Here's how the part is built. I have some questions about the finished solid (model axes, mm). A direction names the side the tool comes from. Round coordinates to 2 decimals unless told otherwise and drop trailing zeros. Order: outer loops, then holes, each group sorted by start corner. A loop starts at its lowest first (then second) coordinate and runs counter-clockwise, first axis right, second up. Notation, with made-up numbers: M 84,27 L 96,27 A22 ccw 96,38 Z; hole C 45.25,-25 d8. An arc over 180 degrees is marked long. Write each question's results on one line, items separated by ' | '. Start each with the question number.
```python
from build123d import *

# Parameters (mm, degrees)
F1_DEPTH = 12.7
F3_DEPTH = 25.4
F4_R     = 1.685949
F5_DEPTH = 25.4


with BuildPart() as f1:
    # F0 (on Front) → F1 (new body)
    with BuildSketch(Plane.XZ):
        Polygon((6.618203, -46.038546), (-16.379258, 0), (-39.209124, -45.537699), (-89.660898, -53.551219), (-53.232785, -89.361645), (-61.747152, -139.553732), (-16.671093, -115.906432), (28.655386, -139.553732), (20.14102, -89.361645), (56.902383, -53.551219), align=None)
    extrude(amount=F1_DEPTH)

    # F2 (on face) → F3 (cut)
    with BuildSketch(Plane.XZ.offset(12.7)):
        Polygon((3.150909, -52.012134), (-16.268918, -10.524325), (-34.585346, -52.012134), (-70.335478, -56.646414), (-44.074576, -82.686633), (-51.136333, -121.526286), (-16.379258, -103.871897), (18.819179, -126.60192), (10.654025, -86.879551), (38.901042, -59.073891), align=None)
    extrude(amount=-F3_DEPTH, mode=Mode.SUBTRACT)

    # F4 (on face) → F5 (cut)
    with BuildSketch(Plane.XZ.offset(12.7)):
        with Locations((-80.045395, -56.205053)):
            Circle(F4_R)
    extrude(amount=-F5_DEPTH, mode=Mode.SUBTRACT)


solid = f1.part
```
(1) I want a section at D-D on x = 42.5. Write out the boundary of the cut face in (y, z), and give its area (3 significant figures).
(2) I want a section at A-A on z = -19. Write out the boundary of the cut face in (x, y), and give its area (3 significant figures).
(3) I'm going to push flat-ended pins straight in: pin 1 Ø6 at (y, z) = (-8.5, -120) entering from -X; pin 2 Ø4 at (y, z) = (-11, -14) entering from +X; pin 3 Ø4 at (x, y) = (-43, -11) entering from -Z. Where does each tip first touch, or does it pass through?
(4) I want a section at C-C on z = -123.5. Write out the boundary of the cut face in (x, y).
(5) Please list where these lines run through material, in increasing order: line 1 (Z direction, x = -25, y = -7.75); line 2 (X direction, y = -9.5, z = -109); line 3 (X direction, y = -7, z = -68).
(6) If we mould it in two halves opening along X, with no side actions, what happens to faces 4 (the cylindrical face through (-81.29, -6.44, -55.07)), 5 (the flat face through (-64.08, -6.26, -49.49)), 6 (the flat face through (-4.72, -6.26, -23.34))? For each: pulls with the +X half, pulls with the -X half, needs draft (parallel to the pull), parting line crosses it, or undercut.
(7) I want a section at B-B on y = -11. Write out the boundary of the cut face in (x, z).
(8) On a 3-axis mill with a long thin cutter (end or side, diameter ignored), from which of +Z, -Z, +X, -X, +Y, -Y can I reach the whole of each face in a straight line? I mean faces 1 (the flat face through (5.67, -6.26, -127.56)), 2 (the flat face through (0.974, -6.439, -115.078)), 3 (the flat face through (38.26, -6.26, -71.71)). Say none if no direction works.
Solutions:
1) outline: M -12.7,-67.58 L 0,-67.58 L 0,-51.4 L -12.7,-51.4 Z | area: 206 mm^2
2) outline: M -25.9,-12.7 L -20.01,-12.7 L -20.01,0 L -25.9,0 Z; M -12.3,-12.7 L -6.89,-12.7 L -6.89,0 L -12.3,0 Z | area: 144 mm^2
3) pin 1: x = -58.94 | pin 2: x = -8.39 | pin 3: z = -130.77
4) outline: M -59.02,-12.7 L -31.15,-12.7 L -31.15,0 L -59.02,0 Z; M -2.12,-12.7 L 14.02,-12.7 L 14.02,0 L -2.12,0 Z; M 18.18,-12.7 L 25.93,-12.7 L 25.93,0 L 18.18,0 Z
5) line 1: -120.28 to -108.25, -30.3 to -17.2 | line 2: -56.56 to -48.86, -26.48 to -8.44, 15.2 to 23.47 | line 3: -74.96 to -58.89, 29.83 to 42.07
6) face 4: undercut | face 5: pulls with the -X half | face 6: pulls with the +X half
7) outline: M -89.66,-53.55 L -53.23,-89.36 L -61.75,-139.55 L -16.67,-115.91 L 28.66,-139.55 L 20.14,-89.36 L 56.9,-53.55 L 6.62,-46.04 L -16.38,0 L -39.21,-45.54 Z; hole C -80.05,-56.21 d3.37; hole M -70.34,-56.65 L -44.07,-82.69 L -51.14,-121.53 L -16.38,-103.87 L 18.82,-126.6 L 10.65,-86.88 L 38.9,-59.07 L 3.15,-52.01 L -16.27,-10.52 L -34.59,-52.01 Z
8) face 1: -Z, +Y, -Y | face 2: +Y, -Y | face 3: +X, +Y, -Y
